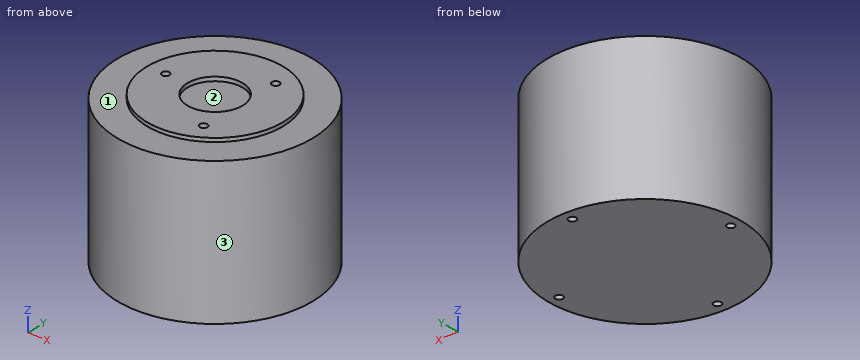
```python
from build123d import *

# Parameters (mm, degrees)
F_0000_CYLINDER_SKETCH_R = 26.5
F_0000_CYLINDER_DEPTH    = 39.2
F_0002_CYLINDER_SKETCH_R = 18.5
F_0002_CYLINDER_DEPTH    = 1.5
F_0004_CYLINDER_SKETCH_R = 7.5
F_0004_CYLINDER_DEPTH    = 1.1
F_0006_CYLINDER_SKETCH_R = 1.025
F_0006_CYLINDER_DEPTH    = 3
F_0009_CYLINDER_SKETCH_R = 1.025
F_0009_CYLINDER_DEPTH    = 3
F_0012_CYLINDER_SKETCH_R = 1.025
F_0012_CYLINDER_DEPTH    = 3
F_0015_CYLINDER_SKETCH_R = 1.025
F_0015_CYLINDER_DEPTH    = 5
F_0018_CYLINDER_SKETCH_R = 1.025
F_0018_CYLINDER_DEPTH    = 5
F_0021_CYLINDER_SKETCH_R = 1.025
F_0021_CYLINDER_DEPTH    = 5
F_0024_CYLINDER_SKETCH_R = 1.025
F_0024_CYLINDER_DEPTH    = 5


with BuildPart() as part:
    # 0000_cylinder_Sketch → 0000_cylinder (new body)
    with BuildSketch(Plane.XY):
        Circle(F_0000_CYLINDER_SKETCH_R)
    extrude(amount=F_0000_CYLINDER_DEPTH)


with BuildPart() as part_1:
    # 0000_cylinder_Translate: moved
    add(part.part.moved(Location((0, 0, -40.2))))


with BuildPart() as body_2:
    # 0002_cylinder_Sketch → 0002_cylinder (new body)
    with BuildSketch(Plane.XY):
        Circle(F_0002_CYLINDER_SKETCH_R)
    extrude(amount=F_0002_CYLINDER_DEPTH)


with BuildPart() as body_2_1:
    # 0002_cylinder_Translate: moved
    add(body_2.part.moved(Location((0, 0, -1.5))))


with BuildPart() as part_2:
    add(part_1.part)

    # 0003_add: union body 2
    add(body_2_1.part)


with BuildPart() as body_2_2:
    # 0004_cylinder_Sketch → 0004_cylinder (new body)
    with BuildSketch(Plane.XY):
        Circle(F_0004_CYLINDER_SKETCH_R)
    extrude(amount=F_0004_CYLINDER_DEPTH)


with BuildPart() as body_2_2_1:
    # 0004_cylinder_Translate: moved
    add(body_2_2.part.moved(Location((0, 0, -1.1))))


with BuildPart() as part_3:
    add(part_2.part)

    # 0005_sub: cut body 2 2
    add(body_2_2_1.part, mode=Mode.SUBTRACT)


with BuildPart() as body_2_3:
    # 0006_cylinder_Sketch → 0006_cylinder (new body)
    with BuildSketch(Plane.XY):
        Circle(F_0006_CYLINDER_SKETCH_R)
    extrude(amount=F_0006_CYLINDER_DEPTH)


with BuildPart() as body_2_3_1:
    # 0006_cylinder_Translate: moved
    add(body_2_3.part.moved(Location((6.75, 11.691342951, -3))))


with BuildPart() as part_4:
    add(part_3.part)

    # 0008_sub: cut body 2 3
    add(body_2_3_1.part, mode=Mode.SUBTRACT)


with BuildPart() as body_2_4:
    # 0009_cylinder_Sketch → 0009_cylinder (new body)
    with BuildSketch(Plane.XY):
        Circle(F_0009_CYLINDER_SKETCH_R)
    extrude(amount=F_0009_CYLINDER_DEPTH)


with BuildPart() as body_2_4_1:
    # 0009_cylinder_Translate: moved
    add(body_2_4.part.moved(Location((6.75, -11.691342951, -3))))


with BuildPart() as part_5:
    add(part_4.part)

    # 0011_sub: cut body 2 4
    add(body_2_4_1.part, mode=Mode.SUBTRACT)


with BuildPart() as body_2_5:
    # 0012_cylinder_Sketch → 0012_cylinder (new body)
    with BuildSketch(Plane.XY):
        Circle(F_0012_CYLINDER_SKETCH_R)
    extrude(amount=F_0012_CYLINDER_DEPTH)


with BuildPart() as body_2_5_1:
    # 0012_cylinder_Translate: moved
    add(body_2_5.part.moved(Location((-13.5, 0, -3))))


with BuildPart() as part_6:
    add(part_5.part)

    # 0014_sub: cut body 2 5
    add(body_2_5_1.part, mode=Mode.SUBTRACT)


with BuildPart() as body_2_6:
    # 0015_cylinder_Sketch → 0015_cylinder (new body)
    with BuildSketch(Plane.XY):
        Circle(F_0015_CYLINDER_SKETCH_R)
    extrude(amount=F_0015_CYLINDER_DEPTH)


with BuildPart() as body_2_6_1:
    # 0015_cylinder_Translate: moved
    add(body_2_6.part.moved(Location((0, 23.5, -40.2))))


with BuildPart() as part_7:
    add(part_6.part)

    # 0017_sub: cut body 2 6
    add(body_2_6_1.part, mode=Mode.SUBTRACT)


with BuildPart() as body_2_7:
    # 0018_cylinder_Sketch → 0018_cylinder (new body)
    with BuildSketch(Plane.XY):
        Circle(F_0018_CYLINDER_SKETCH_R)
    extrude(amount=F_0018_CYLINDER_DEPTH)


with BuildPart() as body_2_7_1:
    # 0018_cylinder_Translate: moved
    add(body_2_7.part.moved(Location((23.5, 0, -40.2))))


with BuildPart() as part_8:
    add(part_7.part)

    # 0020_sub: cut body 2 7
    add(body_2_7_1.part, mode=Mode.SUBTRACT)


with BuildPart() as body_2_8:
    # 0021_cylinder_Sketch → 0021_cylinder (new body)
    with BuildSketch(Plane.XY):
        Circle(F_0021_CYLINDER_SKETCH_R)
    extrude(amount=F_0021_CYLINDER_DEPTH)


with BuildPart() as body_2_8_1:
    # 0021_cylinder_Translate: moved
    add(body_2_8.part.moved(Location((0, -23.5, -40.2))))


with BuildPart() as part_9:
    add(part_8.part)

    # 0023_sub: cut body 2 8
    add(body_2_8_1.part, mode=Mode.SUBTRACT)


with BuildPart() as body_2_9:
    # 0024_cylinder_Sketch → 0024_cylinder (new body)
    with BuildSketch(Plane.XY):
        Circle(F_0024_CYLINDER_SKETCH_R)
    extrude(amount=F_0024_CYLINDER_DEPTH)


with BuildPart() as body_2_9_1:
    # 0024_cylinder_Translate: moved
    add(body_2_9.part.moved(Location((-23.5, 0, -40.2))))


with BuildPart() as part_10:
    add(part_9.part)

    # 0026_sub: cut body 2 9
    add(body_2_9_1.part, mode=Mode.SUBTRACT)


solid = part_10.part
```
Geometry check sheet. Reference: the model listing, model coordinates, mm. Face numbers are marked on the shaded views. Give positions to 0.01 mm unless a question says otherwise; leave off trailing zeros. Order: outer loops, then holes, each group sorted by start corner. A loop starts at its lowest first (then second) coordinate and runs counter-clockwise, first axis right, second up. Notation, with made-up numbers: (63.5, -31) -> (88.5, -31) arc R35 ccw to (88.5, 7) -> close; hole circle Ø3 at (11.25, 71). An arc over 180 degrees is marked (long way). Write each question's results on one line, items separated by ' | '. Start each with the question number.
(1) Sectioned sample at B-B (x = 0). Enter the section's corners in (y, z) (3 decimals).
(2) Sectioned sample at D-D (x = -16). Enter the section's corners in (y, z), plus the area to 3 significant figures.
(3) Gauge pin test, flat ends, axial feed: P1, Ø1.2, axis at x = -23.5, y = 0, coming from the -Z side; P2, Ø8, axis at y = 4.5, z = -34.5, coming from the -X side; P3, Ø0.6, axis at x = 7, y = 11.5, coming from the +Z side. Record the tip position at first contact, or that the pin passes through.
(4) Scan lines: line 1 (Z direction, x = 9.5, y = 18); line 2 (X direction, y = 0.5, z = -31.5); line 3 (Z direction, x = -0.5, y = 24). Record each from-to range of solid material in increasing order.
(5) Sectioned sample at A-A (y = 0). Enter the section's corners in (x, z) (3 decimals).
(6) Mould release check, pull along X, two halves, no side actions. Record for the marked faces 1, 2 and 3: pulls with the +X half, pulls with the -X half, needs draft (parallel to the pull), parting line crosses it, or undercut.
(7) Sectioned sample at C-C (z = -4). Enter the section's corners in (x, y).
Answer below:
1) outline: (-26.5, -40.2) -> (-24.525, -40.2) -> (-24.525, -35.2) -> (-22.475, -35.2) -> (-22.475, -40.2) -> (22.475, -40.2) -> (22.475, -35.2) -> (24.525, -35.2) -> (24.525, -40.2) -> (26.5, -40.2) -> (26.5, -1) -> (18.5, -1) -> (18.5, 0) -> (7.5, 0) -> (7.5, -1.1) -> (-7.5, -1.1) -> (-7.5, 0) -> (-18.5, 0) -> (-18.5, -1) -> (-26.5, -1) -> close
2) outline: (-21.12, -40.2) -> (21.12, -40.2) -> (21.12, -1) -> (9.29, -1) -> (9.29, 0) -> (-9.29, 0) -> (-9.29, -1) -> (-21.12, -1) -> close | area: 1,670 mm2
3) P1: z = -35.2 | P2: x = -26.5 | P3: z = -3
4) line 1: -40.2 to -1 | line 2: -26.5 to 26.5 | line 3: -35.2 to -1
5) outline: (-26.5, -40.2) -> (-24.525, -40.2) -> (-24.525, -35.2) -> (-22.475, -35.2) -> (-22.475, -40.2) -> (22.475, -40.2) -> (22.475, -35.2) -> (24.525, -35.2) -> (24.525, -40.2) -> (26.5, -40.2) -> (26.5, -1) -> (18.5, -1) -> (18.5, 0) -> (7.5, 0) -> (7.5, -1.1) -> (-7.5, -1.1) -> (-7.5, 0) -> (-12.475, 0) -> (-12.475, -3) -> (-14.525, -3) -> (-14.525, 0) -> (-18.5, 0) -> (-18.5, -1) -> (-26.5, -1) -> close
6) face 1: needs draft | face 2: undercut | face 3: parting line crosses it
7) outline: circle Ø53 at (0, 0)
